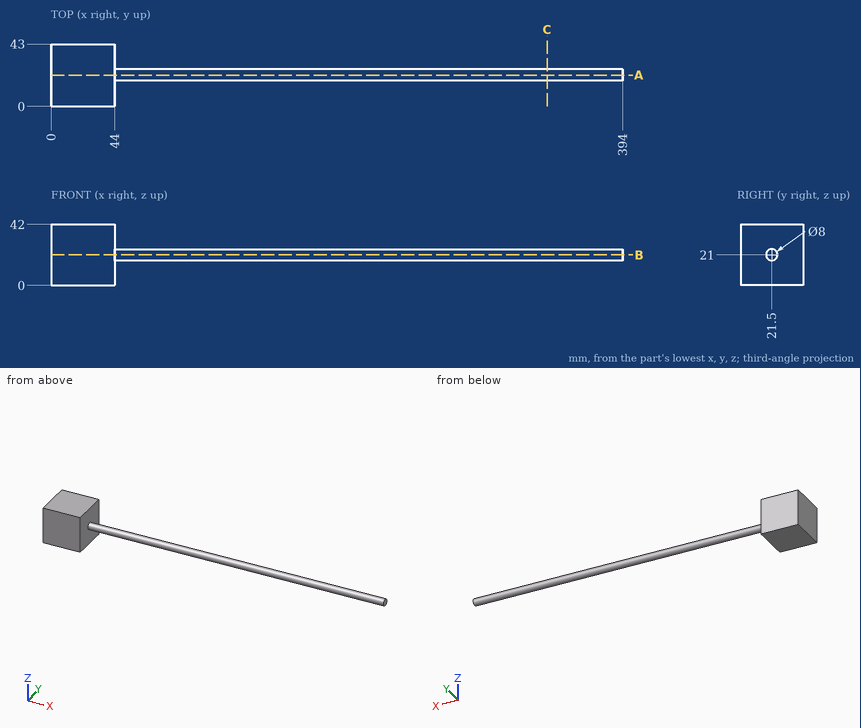
Study the drawing (mm; zero at the part's minimum x, y, z) and answer. Coordinates: 2 decimals unless noted, no trailing zeros. Write each loop counter-clockwise with the first axis right and the second up, starting at its lowest first coordinate (ties: lowest second). Pieces come first, ordered by that corner, then holes.
Q1. Section A-A, the plane y = 21.5 is taken. Write down the section's boundary in (x, z).
Returned:
outline: (0, 0) - (44, 0) - (44, 17) - (394, 17) - (394, 25) - (44, 25) - (44, 42) - (0, 42) - close
Q2. Section C-C, the plane x = 342 is taken. Write down the section's boundary in (y, z).
Returned:
outline: circle Ø8 at (21.5, 21)
Q3. Given P1, Ø8, axis at x = 103.5, y = 20.5, coming from the -Z side; P2, Ø3, axis at x = 140.5, z = 23.5, coming from the -Y side, each flat-ended and moving along its own axis, determine where each tip first touches the part or whether it passes through.
Returned:
P1: stops at z = 17
P2: stops at y = 17.63
Q4. Section B-B, the plane z = 21 is taken. Write down the section's boundary in (x, y).
Returned:
outline: (0, 0) - (44, 0) - (44, 17.5) - (394, 17.5) - (394, 25.5) - (44, 25.5) - (44, 43) - (0, 43) - close
Q5. Find the intervals of material crossed by line 1 along X through (y, z) = (33, 39); line 2 along Z through (x, y) = (299, 20); line 3 along Y through (x, z) = (306, 18), in increasing order.
Returned:
line 1: x = 0 to 44
line 2: z = 17.29 to 24.71
line 3: y = 18.85 to 24.15
